```python
from build123d import *

# Parameters (mm, degrees)
CYLINDER_R        = 2.4
CYLINDER_DEPTH    = 10
ARRAY_X_COUNT     = 2
ARRAY_X_PITCH     = 29.2
ARRAY_Y_COUNT     = 2
ARRAY_Y_PITCH     = 29.2
BOX_W             = 40
BOX_H             = 40
BOX_DEPTH         = 4
FILLET_R          = 2
TORUS_R           = 1.5
CYLINDER001_R     = 17
CYLINDER001_DEPTH = 50
FILLET001_R       = 2


with BuildPart() as taladros_vector:
    # Cylinder → Cylinder (new body)
    with BuildSketch(Plane(origin=(5.4, 5.4, 0), x_dir=(1, 0, 0), z_dir=(0, 0, 1))):
        Circle(CYLINDER_R)
    extrude(amount=CYLINDER_DEPTH)

    # Array X: taladros_vector ×2


with BuildPart() as taladros_vector_1:
    add(taladros_vector.part)
    with Locations(*[(i * ARRAY_X_PITCH, 0, 0) for i in range(1, ARRAY_X_COUNT)]):
        add(taladros_vector.part)

    # Array Y: taladros_vector ×2


with BuildPart() as taladros_vector_2:
    add(taladros_vector_1.part)
    with Locations(*[(0, i * ARRAY_Y_PITCH, 0) for i in range(1, ARRAY_Y_COUNT)]):
        add(taladros_vector_1.part)


with BuildPart() as taladros_vector_3:
    # Array placement: moved
    add(taladros_vector_2.part.moved(Location((0, 0, -3))))


with BuildPart() as obj1:
    # Box → Box (new body)
    with BuildSketch(Plane.XY):
        with Locations((20, 20)):
            Rectangle(BOX_W, BOX_H)
    extrude(amount=BOX_DEPTH)

    # Fillet
    fillet_edges = [obj1.edges().sort_by_distance(p)[0] for p in [
        (0, 0, 2),
        (0, 40, 2),
        (40, 0, 2),
        (40, 40, 2),
    ]]
    fillet(fillet_edges, radius=FILLET_R)

    # Cut: cut taladros_vector
    add(taladros_vector_3.part, mode=Mode.SUBTRACT)


with BuildPart() as obj2:
    # Torus → Torus (revolve)
    with BuildSketch(Plane(origin=(0, 0, 50), x_dir=(1, 0, 0), z_dir=(0, -1, 0))):
        with Locations((10.5, 0)):
            Circle(TORUS_R)
    revolve(axis=Axis((0, 0, 50), (0, 0, 1)))


with BuildPart() as obj3:
    # Cylinder001 → Cylinder001 (new body)
    with BuildSketch(Plane.XY):
        Circle(CYLINDER001_R)
    extrude(amount=CYLINDER001_DEPTH)

    # Fillet001
    fillet001_edges = [obj3.edges().sort_by_distance(p)[0] for p in [
        (-17, 0, 50),
    ]]
    fillet(fillet001_edges, radius=FILLET001_R)

    # Cut001: cut obj2
    add(obj2.part, mode=Mode.SUBTRACT)


with BuildPart() as obj3_1:
    # Cut001 placement: moved
    add(obj3.part.moved(Location((20, 20, 0))))

    # Fusion: union obj1
    add(obj1.part)


solid = obj3_1.part
```
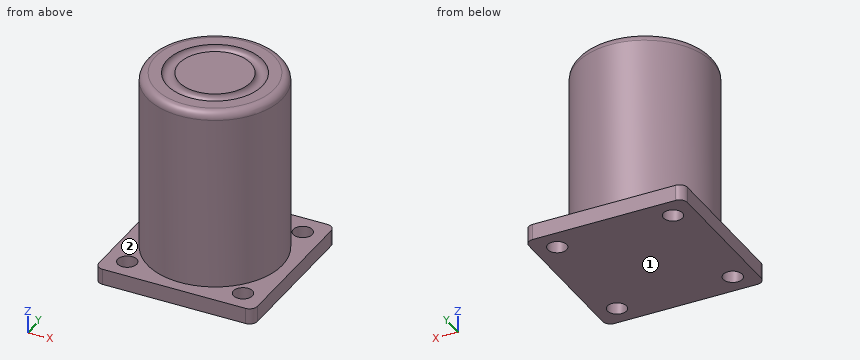
The model under review builds one solid part; all positions refer to its coordinate system, in mm. Face numbers are marked on the shaded views. A direction names the side the tool comes from. Round coordinates to 2 decimals unless told otherwise and drop trailing zeros. Loops run counter-clockwise (first coordinate to the right, second up) from the corner with the lowest first, then second, coordinate; pieces in that order, holes last.
1) Consider section C-C on x = 33. Give the number of separate pieces and of enclosed holes in the cut face, then the cut area to 3 significant figures.
Values follow:
separate pieces: 3
enclosed holes: 0
area: 1,140 mm2
2) Consider section B-B on z = 5. State the section outline as (x, y) points.
Values follow:
outline: circle Ø34 at (20, 20)
3) Clearance check with flat-ended pins moving along their axes: P1, Ø6, axis at x = 31.5, z = 36, coming from the +Y side; P2, Ø4, axis at x = 32, z = 31.5, coming from the +Y side; P3, Ø4, axis at x = 5.4, y = 5.4, coming from the +Z side; P4, Ø7.5, axis at x = 5.4, y = 34.6, coming from the -Z side. State where each tip first meets the part, or that it passes through.
Values follow:
P1: stops at y = 34.72
P2: stops at y = 33.75
P3: passes through
P4: stops at z = 0
4) Consider section A-A on x = 20. State the section outline as (y, z) points, then the cut area to 3 significant figures.
Values follow:
outline: (0, 0) - (40, 0) - (40, 4) - (37, 4) - (37, 48) arc R2 ccw to (35, 50) - (32, 50) arc R1.5 cw to (29, 50) - (11, 50) arc R1.5 cw to (8, 50) - (5, 50) arc R2 ccw to (3, 48) - (3, 4) - (0, 4) - close
area: 1,720 mm2
5) Wall thickness on line 1 along Y through (x, z) = (5.4, 2.65); line 2 along X through (y, z) = (34, 2): over which ranges is each line inside the solid? List them lowest first.
Values follow:
line 1: y = 0 to 3, 7.8 to 32.2, 37 to 40
line 2: x = 0 to 3.08, 7.72 to 32.28, 36.92 to 40
6) Tool access review of the marked faces 1 and 2: name each direction out of +Z, -Z, +X, -X, +Y, -Y from which nothing blocks a thin tool from reaching the whole face with its end or side.
Values follow:
face 1: -Z, +X, -X, +Y, -Y
face 2: +Z
